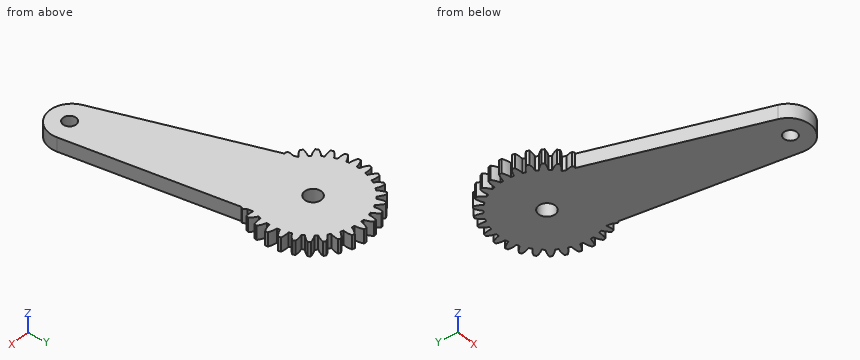
```python
from build123d import *

# Parameters (mm, degrees)
SKETCH1_R           = 12.8
BOSS_EXTRUDE1_DEPTH = 3.18
CUT_EXTRUDE1_DEPTH  = 19.379129468
CIRPATTERN1_COUNT   = 30
SKETCH4_R           = 1.875
CUT_EXTRUDE3_DEPTH  = 19.349437359
BOSS_EXTRUDE2_START = -3.18
BOSS_EXTRUDE2_DEPTH = 3.18
SKETCH7_R           = 1.47
CUT_EXTRUDE4_DEPTH  = 53.659533455


with BuildPart() as part:
    # Sketch1 → Boss-Extrude1 (new body)
    with BuildSketch(Plane.XY):
        with Locations(Location((0, 0, 0), (0, 0, 180))):
            Circle(SKETCH1_R)
    extrude(amount=BOSS_EXTRUDE1_DEPTH)

    # Sketch2 → Cut-Extrude1 (cut, through all)
    with BuildSketch(Plane.XY.offset(3.18)):
        with BuildLine():
            ThreePointArc((-0.321034752, 10.995314306), (0, 11), (0.321034752, 10.995314306))
            ThreePointArc((0.321034752, 10.995314306), (0.594388904, 11.912556329), (1.044293354, 12.75732932))
            ThreePointArc((1.044293354, 12.75732932), (0, 12.8), (-1.044293354, 12.75732932))
            ThreePointArc((-1.044293354, 12.75732932), (-0.594388904, 11.912556329), (-0.321034752, 10.995314306))
        make_face()
    cut_extrude1 = extrude(amount=-CUT_EXTRUDE1_DEPTH, mode=Mode.SUBTRACT)

    # CirPattern1: Cut-Extrude1 ×30 about axis
    cirpattern1_axis = Axis((0, 0, 0), (0, 0, 1))
    for i in range(1, CIRPATTERN1_COUNT):
        add(cut_extrude1.rotate(cirpattern1_axis, i * 360 / CIRPATTERN1_COUNT), mode=Mode.SUBTRACT)

    # Sketch4 → Cut-Extrude3 (cut, through all)
    with BuildSketch(Plane(origin=(0, 0, 0), x_dir=(-1, 0, 0), z_dir=(0, 0, -1))):
        Circle(SKETCH4_R)
    extrude(amount=-CUT_EXTRUDE3_DEPTH, mode=Mode.SUBTRACT)

    # Sketch6 → Boss-Extrude2 (add)
    with BuildSketch(Plane(origin=(0, 0, 0), x_dir=(-1, 0, 0), z_dir=(0, 0, -1)).offset(BOSS_EXTRUDE2_START)):
        with BuildLine():
            Line((-9.828614264, -4.939467749), (-15.386321044, -44.551484806))
            ThreePointArc((-15.386321044, -44.551484806), (-11.558440512, -50.118310067), (-5.67917693, -46.790176566))
            Line((-5.67917693, -46.790176566), (6.672650371, -8.74504071))
            ThreePointArc((6.672650371, -8.74504071), (-2.471967519, -10.71864621), (-9.828614264, -4.939467749))
        make_face()
    extrude(amount=BOSS_EXTRUDE2_DEPTH)

    # Sketch7 → Cut-Extrude4 (cut, through all)
    with BuildSketch(Plane.XY.offset(3.18)):
        with Locations((10.532748987, -45.670830686)):
            Circle(SKETCH7_R)
    extrude(amount=-CUT_EXTRUDE4_DEPTH, mode=Mode.SUBTRACT)


solid = part.part
```
Could you check a few things on this model? Use its own coordinates, in mm. Give positions to 0.01 mm unless a question says otherwise; leave off trailing zeros. Loops run counter-clockwise (first coordinate to the right, second up) from the corner with the lowest first, then second, coordinate; pieces in that order, holes last. Notation, with made-up numbers: (15, -16) - (25, -16) arc R12 cw to (25, 0) - close; hole circle Ø10 at (-21, -15). An arc over 180 degrees is marked (long way). Answer in a Markdown table with one row per item. Add a question column.
Q1. For pin 1 (1.5 mm diameter, centred on y = -29, z = 1.5, fed in from -X); pin 2 (4 mm diameter, centred on x = 8, y = -16, fed in from -Z), each with a flat end and sliding along its axis, tell me the tip position at first contact or that it passes through.
Q2. If we section it at A-A (z = 1.05): State how many separate pieces and enclosed holes the cut face has, plus the area to 3 significant figures.
Q3. Please list where these lines run through material, in increasing order: L1, parallel to X at y = -13, z = 2.4; L2, parallel to Y at x = 9.25, z = 3; L3, parallel to X at y = -10.5, z = 2.6. Write a range as from..to.
Q4. If we section it at C-C (y = -30.5): List the corners of the cut face in (x, z) for me, plus the area to 3 significant figures.
Q5. If we section it at B-B (y = -19): List the corners of the cut face in (x, z) for me, plus the area to 3 significant figures.
The answers:
| question | item | result |
|---|---|---|
| 1 | pin 1 | stops at x = -0.34 |
| 1 | pin 2 | stops at z = 0 |
| 2 | separate pieces | 1 |
| 2 | enclosed holes | 2 |
| 2 | area | 937 mm^2 |
| 3 | L1 | x = -5.29..10.96 |
| 3 | L2 | y = -50.1..-46.39, -44.95..7.53 |
| 3 | L3 | x = -6.62..10.61 |
| 4 | outline | (0.39, 0) - (13.41, 0) - (13.41, 3.18) - (0.39, 3.18) - close |
| 4 | area | 41.4 mm^2 |
| 5 | outline | (-3.34, 0) - (11.8, 0) - (11.8, 3.18) - (-3.34, 3.18) - close |
| 5 | area | 48.2 mm^2 |
